Can you work these out from the model? Positions are in its coordinate system, mm. Face numbers are marked on the shaded views. A direction names the side the tool comes from. Coordinates: 2 decimals unless noted, no trailing zeros. Loops run counter-clockwise (first coordinate to the right, second up) from the corner with the lowest first, then second, coordinate; pieces in that order, holes last.
```python
from build123d import *

# Parameters (mm, degrees)
BOSS_EXTRUDE1_DEPTH                                  = 50.8
CBORE_FOR_1_4_BINDING_HEAD_MACHINE_SCREW_D           = 6.5278
CBORE_FOR_1_4_BINDING_HEAD_MACHINE_SCREW_CBORE_D     = 14.2875
CBORE_FOR_1_4_BINDING_HEAD_MACHINE_SCREW_CBORE_DEPTH = 4.064
CUT_EXTRUDE1_REACH                                   = 73.2
SKETCH4_R                                            = 4.9022


with BuildPart() as part:
    # Sketch1 → Boss-Extrude1 (new body)
    with BuildSketch(Plane(origin=(0, 0, 0), x_dir=(0, 0, -1), z_dir=(1, 0, 0))):
        Polygon((0, 0), (0, 31.75), (38.480114202, 31.75), (38.480114202, 26.2001), (7.62, 26.2001), (7.62, 5.5499), (38.480114202, 5.5499), (38.480114202, 0), align=None)
    extrude(amount=BOSS_EXTRUDE1_DEPTH)

    # CBORE for 1/4 Binding Head Machine Screw1 (through all)
    with Locations(Plane(origin=(0, 0, -7.62), x_dir=(-1, 0, 0), z_dir=(0, 0, -1))):
        with Locations((-12.7, 15.875), (-38.1, 15.875)):
            CounterBoreHole(CBORE_FOR_1_4_BINDING_HEAD_MACHINE_SCREW_D / 2, CBORE_FOR_1_4_BINDING_HEAD_MACHINE_SCREW_CBORE_D / 2, CBORE_FOR_1_4_BINDING_HEAD_MACHINE_SCREW_CBORE_DEPTH)

    # Cut-Extrude1: up to this face of the body (flat: up to its plane)
    cut_extrude1_end = Plane(part.part.faces().sort_by_distance((25.4, 31.75, -19.240057101))[0])
    # Sketch4 → Cut-Extrude1 (cut, up to the picked face)
    with BuildSketch(Plane.XZ, mode=Mode.PRIVATE) as cut_extrude1_sk1:
        with Locations(Location((25.4, -25.780114202, 0), (0, 0, 270))):
            Circle(SKETCH4_R)
    cut_extrude1_tool1 = split(extrude(cut_extrude1_sk1.sketch, amount=-CUT_EXTRUDE1_REACH, mode=Mode.PRIVATE), bisect_by=cut_extrude1_end, keep=Keep.BOTH, mode=Mode.PRIVATE)
    # Sketch4 → Cut-Extrude1 (cut, up to the picked face)
    with BuildSketch(Plane.XZ, mode=Mode.PRIVATE) as cut_extrude1_sk2:
        Polygon((19.05, -34.124014202), (0, -6.35), (0, -38.480114202), (50.8, -38.480114202), (50.8, -6.35), (31.75, -34.124014202), align=None)
    cut_extrude1_tool2 = split(extrude(cut_extrude1_sk2.sketch, amount=-CUT_EXTRUDE1_REACH, mode=Mode.PRIVATE), bisect_by=cut_extrude1_end, keep=Keep.BOTH, mode=Mode.PRIVATE)
    add(cut_extrude1_tool1.solids().sort_by(Axis((25.4, 0, -25.780114), (0, 1, 0)))[0], mode=Mode.SUBTRACT)
    add(cut_extrude1_tool2.solids().sort_by(Axis((9.029312, 0, -20.576996), (0, 1, 0)))[0], mode=Mode.SUBTRACT)


solid = part.part
```
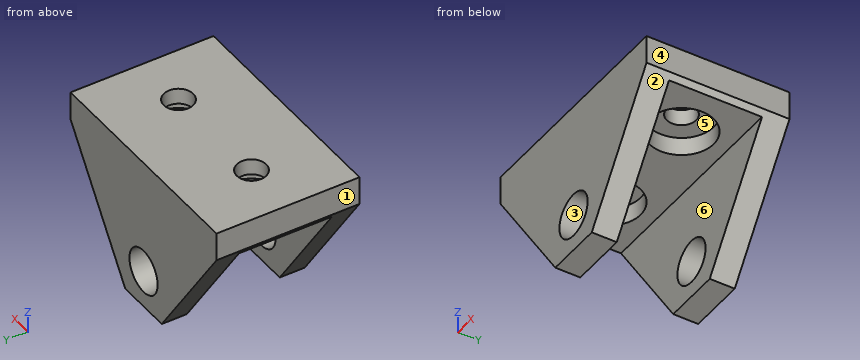
(1) I want a section at B-B on z = -10. Write out the boundary of the cut face in (x, y).
Check values:
outline: (2.5, 0) - (48.3, 0) - (48.3, 5.55) - (2.5, 5.55) - close; (2.5, 26.2) - (48.3, 26.2) - (48.3, 31.75) - (2.5, 31.75) - close
(2) I want a section at D-D on y = 14. Write out the boundary of the cut face in (x, z), then the cut area to 3 significant figures.
Check values:
outline: (0, -6.35) - (0.87, -7.62) - (5.81, -7.62) - (5.81, -3.56) - (10.03, -3.56) - (10.03, 0) - (0, 0) - close; (15.37, -3.56) - (19.59, -3.56) - (19.59, -7.62) - (31.21, -7.62) - (31.21, -3.56) - (35.43, -3.56) - (35.43, 0) - (15.37, 0) - close; (40.77, -3.56) - (44.99, -3.56) - (44.99, -7.62) - (49.93, -7.62) - (50.8, -6.35) - (50.8, 0) - (40.77, 0) - close
area: 236 mm2
(3) I want a section at A-A on x = 25.4. Write out the boundary of the cut face in (y, z).
Check values:
outline: (0, -34.12) - (5.55, -34.12) - (5.55, -30.68) - (0, -30.68) - close; (0, -20.88) - (5.55, -20.88) - (5.55, -7.62) - (26.2, -7.62) - (26.2, -20.88) - (31.75, -20.88) - (31.75, 0) - (0, 0) - close; (26.2, -34.12) - (31.75, -34.12) - (31.75, -30.68) - (26.2, -30.68) - close
(4) If we mould it in two halves opening along X, with no side actions, what happens to the marked faces 1, 2 and 3? For each: released by +X, released by -X, zero draft, split by the parting line, or undercut.
Check values:
face 1: released by -X
face 2: released by +X
face 3: undercut
(5) I want a section at C-C on z = -29. Write out the boundary of the cut face in (x, y).
Check values:
outline: (15.54, 0) - (21.7, 0) - (21.7, 5.55) - (15.54, 5.55) - close; (15.54, 26.2) - (21.7, 26.2) - (21.7, 31.75) - (15.54, 31.75) - close; (29.1, 0) - (35.26, 0) - (35.26, 5.55) - (29.1, 5.55) - close; (29.1, 26.2) - (35.26, 26.2) - (35.26, 31.75) - (29.1, 31.75) - close
(6) If I drill on probe 1 along Y at (x, z) = (38.1, -4.5); probe 2 along Y at (x, z) = (28.5, -11); probe 3 along Z at (x, y) = (20.5, 10.5), over which ranges is the centre line in solid material (lowest first)?
Check values:
probe 1: y = 0 to 8.73, 23.02 to 31.75
probe 2: y = 0 to 5.55, 26.2 to 31.75
probe 3: z = -7.62 to 0
(7) I'm going to push flat-ended pins straight in: pin 1 (5 mm diameter, centred on x = 38.1, y = 15.875, fed in from +Z); pin 2 (10.5 mm diameter, centred on x = 14.5, y = 17, fed in from -Z); pin 3 (4 mm diameter, centred on x = 13, y = 13, fed in from -Z). Where does each tip first touch, or does it pass through?
Check values:
pin 1: passes through
pin 2: stops at z = -7.62
pin 3: stops at z = -3.56
(8) Which directions (+Z, -Z, +X, -X, +Y, -Y) give clear straight access to the entire face, cutting with the end or side of a thin tool? Please do the marked faces 4, 5 and 6.
Check values:
face 4: +Z, -Z, +X, +Y, -Y
face 5: -Z
face 6: -Z, +X, -X
